Can you work these out from the model? Positions are in its coordinate system, mm. Give positions to 0.01 mm unless a question says otherwise; leave off trailing zeros. Loops run counter-clockwise (first coordinate to the right, second up) from the corner with the lowest first, then second, coordinate; pieces in that order, holes last. Notation, with made-up numbers: (37, 79) -> (42, 79) arc R13 cw to (42, 85) -> close; hole circle Ø10 at (8, 16). An arc over 180 degrees is marked (long way). One line per question, with ' | ' between items.
from build123d import *

# Parameters (mm, degrees)
SKETCH_2_R          = 1.6
EXTRUDE_1_DEPTH     = 3
SKETCH_4_W          = 6.5
SKETCH_4_H          = 8
CUT_EXTRUDE_1_DEPTH = 3
SKETCH_6_R          = 1.6
CUT_EXTRUDE_2_DEPTH = 10
CUT_EXTRUDE_START   = -10
CUT_EXTRUDE_3_DEPTH = 10
FILLET_1_R          = 2


with BuildPart() as part:
    # 草图2 → 凸台-拉伸1 (new body)
    with BuildSketch(Plane.XY):
        with BuildLine():
            Line((-162.154590294, 76.5), (-162.154590294, 66.5))
            ThreePointArc((-162.154590294, 66.5), (-143.702317509, 21.952272785), (-99.154590294, 3.5))
            Line((-99.154590294, 3.5), (-88, 3.5))
            Line((-88, 3.5), (-88, -11.5))
            Line((-88, -11.5), (-99.154590294, -11.5))
            ThreePointArc((-99.154590294, -11.5), (-154.308919227, 11.345671067), (-177.154590294, 66.5))
            Line((-177.154590294, 66.5), (-177.154590294, 76.5))
            Line((-177.154590294, 76.5), (-162.154590294, 76.5))
        make_face()
        with Locations((-91.754590294, 1)):
            Circle(SKETCH_2_R, mode=Mode.SUBTRACT)
        with Locations((-99.154590294, 1)):
            Circle(SKETCH_2_R, mode=Mode.SUBTRACT)
        with Locations((-106.910050218, 1.460759219)):
            Circle(SKETCH_2_R, mode=Mode.SUBTRACT)
        with Locations((-114.556398703, 2.836554462)):
            Circle(SKETCH_2_R, mode=Mode.SUBTRACT)
        with Locations((-121.986059394, 5.108029688)):
            Circle(SKETCH_2_R, mode=Mode.SUBTRACT)
        with Locations((-129.094504517, 8.243227549)):
            Circle(SKETCH_2_R, mode=Mode.SUBTRACT)
        with Locations((-135.781725472, 12.198038998)):
            Circle(SKETCH_2_R, mode=Mode.SUBTRACT)
        with Locations((-141.953639856, 16.916823855)):
            Circle(SKETCH_2_R, mode=Mode.SUBTRACT)
        with Locations((-147.523415105, 22.333193613)):
            Circle(SKETCH_2_R, mode=Mode.SUBTRACT)
        with Locations((-152.412690143, 28.370945455)):
            Circle(SKETCH_2_R, mode=Mode.SUBTRACT)
        with Locations((-156.552677837, 34.945134346)):
            Circle(SKETCH_2_R, mode=Mode.SUBTRACT)
        with Locations((-159.885132769, 41.963268131)):
            Circle(SKETCH_2_R, mode=Mode.SUBTRACT)
        with Locations((-162.363170682, 49.326608799)):
            Circle(SKETCH_2_R, mode=Mode.SUBTRACT)
        with Locations((-163.951928103, 56.931561629)):
            Circle(SKETCH_2_R, mode=Mode.SUBTRACT)
        with Locations((-164.62905283, 64.671132664)):
            Circle(SKETCH_2_R, mode=Mode.SUBTRACT)
        with Locations((-164.654590294, 72.371090315)):
            Circle(SKETCH_2_R, mode=Mode.SUBTRACT)
    extrude(amount=EXTRUDE_1_DEPTH)

    # 草图4 → 切除-拉伸1 (cut)
    with BuildSketch(Plane.XY.offset(3)):
        with Locations((-173.904590294, 72.5)):
            Rectangle(SKETCH_4_W, SKETCH_4_H)
    extrude(amount=-CUT_EXTRUDE_1_DEPTH, mode=Mode.SUBTRACT)

    # 草图6 → 切除-拉伸2 (cut)
    with BuildSketch(Plane.XY.offset(3)):
        with Locations((-170.287955794, 46.10283567)):
            Circle(SKETCH_6_R)
        with Locations((-159.021847878, 23.00389133)):
            Circle(SKETCH_6_R)
        with Locations((-114.540055415, -5.882922454)):
            Circle(SKETCH_6_R)
        with Locations((-93.154590294, -7.5)):
            Circle(SKETCH_6_R)
    extrude(amount=-CUT_EXTRUDE_2_DEPTH, mode=Mode.SUBTRACT)

    # 草图8 → 切除-拉伸3 (cut)
    with BuildSketch(Plane.XY.offset(3).offset(CUT_EXTRUDE_START)):
        with BuildLine():
            Line((-88, 3.5), (-99.154590294, 3.5))
            ThreePointArc((-99.154590294, 3.5), (-143.702317509, 21.952272785), (-162.154590294, 66.5))
            Line((-162.154590294, 66.5), (-162.154590294, 76.5))
            Line((-162.154590294, 76.5), (-170.654590294, 76.5))
            Line((-170.654590294, 76.5), (-170.654590294, 68.5))
            Line((-170.654590294, 68.5), (-170.154590294, 68.5))
            Line((-170.154590294, 68.5), (-170.154590294, 66.5))
            ThreePointArc((-170.154590294, 66.5), (-149.359171759, 16.295418536), (-99.154590294, -4.5))
            Line((-99.154590294, -4.5), (-88, -4.5))
            Line((-88, -4.5), (-88, 3.5))
        make_face()
    extrude(amount=CUT_EXTRUDE_3_DEPTH, mode=Mode.SUBTRACT)

    # 圆角1
    fillet_1_edges = [part.edges().sort_by_distance(p)[0] for p in [
        (-177.154590294, 68.5, 1.5),
        (-88, -11.5, 1.5),
        (-88, -4.5, 1.5),
        (-170.154590294, 68.5, 1.5),
    ]]
    fillet(fillet_1_edges, radius=FILLET_1_R - 0.0001)  # a hair under: the kernel refuses the full size


solid = part.part
Q1. If we section it at C-C (y = 27): Write out the boundary of the cut face in (x, z), plus the area to 3 significant figures.
Entries:
outline: (-166.41, 0) -> (-158.15, 0) -> (-158.15, 3) -> (-166.41, 3) -> close | area: 24.8 mm²
Q2. If we section it at A-A (z = 2.15): State how many separate pieces and enclosed holes the cut face has, plus the area to 3 significant figures.
Entries:
separate pieces: 1 | enclosed holes: 4 | area: 876 mm²
Q3. If I drill on probe 1 along Y at (x, z) = (-171, 0.85); probe 2 along X at (y, z) = (42.5, 1.7); probe 3 along X at (y, z) = (4, 1.7), over which ranges is the centre line in solid material (lowest first)? Write a range as from..to.
Entries:
probe 1: 36.13..44.67, 47.54..68.13 | probe 2: -173.37..-165.98 | probe 3: -145.82..-132.84
Q4. If we section it at B-B (x = -114): Write out the boundary of the cut face in (y, z), plus the area to 3 significant figures.
Entries:
outline: (-10.07, 0) -> (-7.39, 0) -> (-7.39, 3) -> (-10.07, 3) -> close; (-4.38, 0) -> (-2.93, 0) -> (-2.93, 3) -> (-4.38, 3) -> close | area: 12.4 mm²
Q5. If we mould it in two halves opening along X, with no side actions, what happens to faces 1 (the face through (-95, -4.5, 1)), 2 (the face through (-160.62, 23.07, 1.52)), 3 (the face through (-153.699, 10.743, 1.479)), 4 (the face through (-170.725, 67.899, 1.521))? For each: pulls with the +X half, pulls with the -X half, needs draft (parallel to the pull), parting line crosses it, or undercut.
Entries:
face 1: needs draft | face 2: undercut | face 3: pulls with the -X half | face 4: pulls with the +X half
Q6. For pin 1 Ø1.5 at (y, z) = (58.5, 2.5) entering from -X; pin 2 Ø3.5 at (x, y) = (-114.54, -5.88) entering from -Z; pin 3 Ø1.5 at (x, z) = (-143.5, 2) entering from +Y, each with a flat end and sliding along its axis, tell me the tip position at first contact or that it passes through.
Entries:
pin 1: x = -176.82 | pin 2: z = 0 | pin 3: y = 11.66
Q7. If we section it at D-D (x = -145): Write out the boundary of the cut face in (y, z), plus the area to 3 significant figures.
Entries:
outline: (3.4, 0) -> (12.29, 0) -> (12.29, 3) -> (3.4, 3) -> close | area: 26.7 mm²
